Autodesk Inventor part; units mm, degrees
ref_plane "o1_XY" through (0, -7.8105, 0) normal (1, 0, 0) x (0, 0, -1)
ref_plane "o1_YZ" through (0, -7.8105, 0) normal (0, 0, -1) x (0, 1, 0)
ref_plane "o1_ZX" through (0, -7.8105, 0) normal (0, 1, 0) x (1, 0, 0)
sketch "Sketch_5" plane through (0, 0, 0) normal (0, 0, 1) x (1, 0, 0)
  line L0 (55.5752, 0) -> (-55.5752, 0)
  line L1 (0, 6.9051) -> (0.263, 6.6421)
  line L2 (0.263, 6.6421) -> (0.635, 6.6421)
  line L3 (0.635, 6.6421) -> (1.27, 7.2771)
  line L4 (1.27, 7.2771) -> (54.3052, 7.2771)
  line L5 (54.3052, 7.2771) -> (54.9402, 6.6421)
  line L6 (54.9402, 6.6421) -> (55.3122, 6.6421)
  line L7 (55.3122, 6.6421) -> (55.5752, 6.9051)
  line L8 (55.5752, 6.9051) -> (54.6698, 7.8105)
  line L9 (54.6698, 7.8105) -> (0.9054, 7.8105)
  line L10 (0.9054, 7.8105) -> (0, 6.9051)
revolve "Revolution1" add sketch "Sketch_5" angle 360 about axis through (55.5752, 0, 0) along (1, 0, 0)
sketch "Sketch_1" plane through (0, 0, 0) normal (0, 0, 1) x (1, 0, 0)
  line L0 (46.0502, 0) -> (46.0502, 7.8105)
  line L1 (46.0502, 7.8105) -> (47.244, 7.8105)
  line L2 (47.244, 7.8105) -> (47.244, 0)
  line L3 (47.244, 0) -> (46.0502, 0)
  line L4 (46.0502, 0) -> (46.0502, 7.8105)
revolve "Revolution2" cut sketch "Sketch_1" angle 360 about axis through (46.0502, 0, 0) along (0, -1, 0)
ref_plane "o1_XY" through (0, -7.8105, 0) normal (1, 0, 0) x (0, 0, -1)
ref_plane "o1_YZ" through (0, -7.8105, 0) normal (0, 0, -1) x (0, 1, 0)
ref_plane "o1_ZX" through (0, -7.8105, 0) normal (0, 1, 0) x (1, 0, 0)
ref_plane "o2_XY" through (0, 7.8105, 0) normal (1, 0, 0) x (0, 0, -1)
ref_plane "o2_YZ" through (0, 7.8105, 0) normal (0, 0, -1) x (0, 1, 0)
ref_plane "o2_ZX" through (0, 7.8105, 0) normal (0, 1, 0) x (1, 0, 0)
ref_plane "t1_XY" through (27.7876, 7.8105, 0) normal (1, 0, 0) x (0, 0, -1)
ref_plane "t1_YZ" through (27.7876, 7.8105, 0) normal (0, 0, -1) x (0, 1, 0)
ref_plane "t1_ZX" through (27.7876, 7.8105, 0) normal (0, 1, 0) x (1, 0, 0)
ref_plane "t2_XY" through (27.7876, 0, -7.8105) normal (1, 0, 0) x (0, 0, -1)
ref_plane "t2_YZ" through (27.7876, 0, -7.8105) normal (0, 0, -1) x (0, 1, 0)
ref_plane "t2_ZX" through (27.7876, 0, -7.8105) normal (0, 1, 0) x (1, 0, 0)
ref_plane "t3_XY" through (27.7876, -7.8105, 0) normal (1, 0, 0) x (0, 0, -1)
ref_plane "t3_YZ" through (27.7876, -7.8105, 0) normal (0, 0, -1) x (0, 1, 0)
ref_plane "t3_ZX" through (27.7876, -7.8105, 0) normal (0, 1, 0) x (1, 0, 0)
ref_plane "t4_XY" through (27.7876, 0, 7.8105) normal (1, 0, 0) x (0, 0, -1)
ref_plane "t4_YZ" through (27.7876, 0, 7.8105) normal (0, 0, -1) x (0, 1, 0)
ref_plane "t4_ZX" through (27.7876, 0, 7.8105) normal (0, 1, 0) x (1, 0, 0)
ref_plane "tube1_XY" through (1.27, 0, 0) normal (1, 0, 0) x (0, 0, -1)
ref_plane "tube1_YZ" through (1.27, 0, 0) normal (0, 0, -1) x (0, 1, 0)
ref_plane "tube1_ZX" through (1.27, 0, 0) normal (0, 1, 0) x (1, 0, 0)
ref_plane "tube2_XY" through (54.3052, 0, 0) normal (1, 0, 0) x (0, 0, -1)
ref_plane "tube2_YZ" through (54.3052, 0, 0) normal (0, 0, -1) x (0, 1, 0)
ref_plane "tube2_ZX" through (54.3052, 0, 0) normal (0, 1, 0) x (1, 0, 0)
properties part number "D-75938XP-2.188" material "Steel"
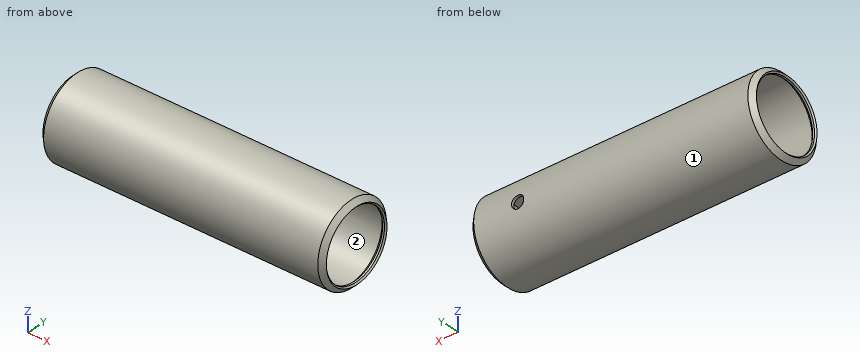
Input: part model. Units: mm. Frame: model coordinates. Face numbers are marked on the shaded views. Coordinates: 2 decimals unless noted, no trailing zeros. Order: outer loops, then holes, each group sorted by start corner. A loop starts at its lowest first (then second) coordinate and runs counter-clockwise, first axis right, second up. Notation, with made-up numbers: M 34,58 L 49,58 A34 cw 49,92 Z; hole C 65.5,10 d2. An arc over 180 degrees is marked long. One line per question, with ' | ' between items.
Item 1: Draft query along Z for the marked faces 1 and 2. Return one class per face: released by +Z, released by -Z, zero draft, split by the parting line, or undercut.
Geometry results:
face 1: split by the parting line | face 2: undercut
Item 2: Section B-B (z = 0). Give the number of separate pieces and of enclosed holes in the cut face, then the cut area to 3 significant figures.
Geometry results:
separate pieces: 3 | enclosed holes: 0 | area: 58.7 mm^2
Item 3: Ray query, line 1 along Z through (x, y) = (44, 0); line 2 along Z through (x, y) = (55.2, 0); line 3 along Y through (x, z) = (36, -0.25). Return the intervals inside material, ascending.
Geometry results:
line 1: z = -7.81 to -7.28, 7.28 to 7.81 | line 2: z = -7.28 to -6.64, 6.64 to 7.28 | line 3: y = -7.81 to -7.27, 7.27 to 7.81
Item 4: Pin query (flat end, axial travel): pin 1 (5 mm diameter, centred on y = -4.5, z = 3, fed in from +X); pin 2 (1.5 mm diameter, centred on y = 0, z = -5.5, fed in from -X); pin 3 (1 mm diameter, centred on x = 23, z = -4.5, fed in from +Y); pin 4 (1.5 mm diameter, centred on x = 19.5, z = 1.5, fed in from -Y). Return the tip coordinate at first contact, or that it passes through.
Geometry results:
pin 1: stops at x = 55.58 | pin 2: passes through | pin 3: stops at y = 6.71 | pin 4: stops at y = -7.77
Item 5: Section C-C (x = 35). Output: boundary loops of the cut face in (y, z).
Geometry results:
outline: C 0,0 d15.62; hole C 0,0 d14.55
